from build123d import *

# Parameters (mm, degrees)
SKETCH_1_R      = 2.15
SKETCH_1_R_2    = 1.65
EXTRUDE_1_DEPTH = 3
FILLET_1_R      = 5


with BuildPart() as part:
    # 草图1 → 凸台-拉伸1 (new body)
    with BuildSketch(Plane.XY):
        Polygon((0, 0), (13, 0), (13, -3), (25, -3), (25, 0), (125, 0), (125, -3), (137, -3), (137, 0), (150, 0), (150, 37.6), (137, 37.6), (137, 40.6), (137, 55.6), (125, 55.6), (125, 40.6), (125, 37.6), (25, 37.6), (25, 40.6), (13, 40.6), (13, 37.6), (0, 37.6), align=None)
        with Locations((131, 49.6)):
            Circle(SKETCH_1_R, mode=Mode.SUBTRACT)
        with Locations((6, 32.6)):
            Circle(SKETCH_1_R_2, mode=Mode.SUBTRACT)
        with Locations((6, 5)):
            Circle(SKETCH_1_R_2, mode=Mode.SUBTRACT)
        with Locations(Location((144, 32.6, 0), (0, 0, 180))):
            Circle(SKETCH_1_R_2, mode=Mode.SUBTRACT)
        with Locations(Location((144, 5, 0), (0, 0, 180))):
            Circle(SKETCH_1_R_2, mode=Mode.SUBTRACT)
    extrude(amount=EXTRUDE_1_DEPTH)

    # 圆角1
    fillet_1_edges = [part.edges().sort_by_distance(p)[0] for p in [
        (125, 55.6, 1.5),
        (137, 55.6, 1.5),
    ]]
    fillet(fillet_1_edges, radius=FILLET_1_R)


solid = part.part
Design review of the part built by this model. Coordinates are the model's own, in mm. A direction names the side the tool comes from. Coordinates: 2 decimals unless noted, no trailing zeros. Order: outer loops, then holes, each group sorted by start corner. A loop starts at its lowest first (then second) coordinate and runs counter-clockwise, first axis right, second up. Notation, with made-up numbers: M -19,43 L -3,43 A16 ccw -3,74 Z; hole C 89.5,59.25 d10. An arc over 180 degrees is marked long. Use a Markdown table: item, result.
(1) For faces 1 (the flat face through (125, 44, 1)), 2 (the flat face through (13, 39, 1)), 3 (the flat face through (6, 0, 1)), 4 (the flat face through (144, 37.6, 1)), list the 3-axis set-ups (+Z, -Z, +X, -X, +Y, -Y) from which the entire face can be reached by the end or side of a thin tool; tool diameter is ignored.
Worked answers:
| item | result |
|---|---|
| face 1 | +Z, -Z, +Y |
| face 2 | +Z, -Z, -X, +Y |
| face 3 | +Z, -Z, -X, -Y |
| face 4 | +Z, -Z, +X, +Y |
(2) For P1, Ø0.9, axis at x = 3.5, z = 1.5, coming from the -Y side; P2, Ø0.9, axis at y = -1.5, z = 2, coming from the +X side, all flat-tipped, find the tip position at first contact; note any pin that passes through.
Worked answers:
| item | result |
|---|---|
| P1 | stops at y = 0 |
| P2 | stops at x = 137 |
(3) Add section D-D (x = 20). Give the boundary of the cut face in (y, z), then the cut area to 3 significant figures.
Worked answers:
| item | result |
|---|---|
| outline | M -3,0 L 40.6,0 L 40.6,3 L -3,3 Z |
| area | 131 mm2 |
(4) Draft analysis for pull direction X (two halves, no side actions). For faces 5 (the flat face through (7, 37.6, 1)), 6 (the cylindrical face through (126.43, 54.1, 1.52)), 7 (the flat face through (25, 39, 1)), 8 (the flat face through (137, -2, 1)), state which applies: released by +X, released by -X, zero draft, split by the parting line, or undercut.
Worked answers:
| item | result |
|---|---|
| face 5 | zero draft |
| face 6 | released by -X |
| face 7 | undercut |
| face 8 | released by +X |
(5) Add section B-B (x = 144). Give the boundary of the cut face in (y, z).
Worked answers:
| item | result |
|---|---|
| outline | M 0,0 L 3.35,0 L 3.35,3 L 0,3 Z; M 6.65,0 L 30.95,0 L 30.95,3 L 6.65,3 Z; M 34.25,0 L 37.6,0 L 37.6,3 L 34.25,3 Z |
(6) Add section A-A (z = 1.35). Give the boundary of the cut face in (x, y).
Worked answers:
| item | result |
|---|---|
| outline | M 0,0 L 13,0 L 13,-3 L 25,-3 L 25,0 L 125,0 L 125,-3 L 137,-3 L 137,0 L 150,0 L 150,37.6 L 137,37.6 L 137,50.6 A5 ccw 132,55.6 L 130,55.6 A5 ccw 125,50.6 L 125,37.6 L 25,37.6 L 25,40.6 L 13,40.6 L 13,37.6 L 0,37.6 Z; hole C 6,5 d3.3; hole C 6,32.6 d3.3; hole C 131,49.6 d4.3; hole C 144,5 d3.3; hole C 144,32.6 d3.3 |
(7) Wall thickness on probe 1 along Y at (x, z) = (6, 0.65); probe 2 along Y at (x, z) = (52, 1.35); probe 3 along X at (y, z) = (39.5, 0.85): over which ranges is each line inside the solid? List them lowest first.
Worked answers:
| item | result |
|---|---|
| probe 1 | y = 0 to 3.35, 6.65 to 30.95, 34.25 to 37.6 |
| probe 2 | y = 0 to 37.6 |
| probe 3 | x = 13 to 25, 125 to 137 |
(8) Add section C-C (y = 5). Give the boundary of the cut face in (x, z).
Worked answers:
| item | result |
|---|---|
| outline | M 0,0 L 4.35,0 L 4.35,3 L 0,3 Z; M 7.65,0 L 142.35,0 L 142.35,3 L 7.65,3 Z; M 145.65,0 L 150,0 L 150,3 L 145.65,3 Z |
